Could you check a few things on this model? Use its own coordinates, in mm. Face numbers are marked on the shaded views. A direction names the side the tool comes from. Round coordinates to 2 decimals unless told otherwise and drop trailing zeros. Write each loop counter-clockwise with the first axis right and the second up, starting at its lowest first coordinate (ties: lowest second). Pieces come first, ordered by that corner, then holes. Notation, with made-up numbers: (18.25, 35) - (56.25, 35) arc R38 ccw to (56.25, 74) - close; hole circle Ø11 at (57, -13). An arc over 180 degrees is marked (long way). Write each question's results on one line, items separated by ' | '. Start each with the question number.
(1) Imagine slicing it at A-A on x = 0. Write out the boundary of the cut face in (y, z), then the cut area to 3 significant figures.
(2) Thinking about a two-plate mould opening in Y: for the marked faces 4, 5 and 6, which applies, +Y half, -Y half, draft (parallel to the pull), parting line (faces both ways), or undercut?
(3) Imagine slicing it at D-D on y = 7.5. Write out the boundary of the cut face in (x, z).
(4) For P1, Ø8, axis at y = -4.5, z = 9.5, coming from the -X side; P2, Ø1.5, axis at y = -8.5, z = 7.5, coming from the -X side; P3, Ø2.5, axis at x = -5.3, y = 5.3, coming from the +Z side; P4, Ø1.7, axis at x = 5.3, y = 5.3, coming from the -Z side, each with a flat end and sliding along its axis, tell me the tip position at first contact or that it passes through.
(5) Please list where these lines run through material, in increasing order: line 1 (Y direction, x = 0, z = 9.25); line 2 (X direction, y = 1.5, z = 7.25); line 3 (Y direction, x = 2.5, z = 13). Write a range as [from, to].
(6) Imagine slicing it at C-C on z = 15.25. Write out the boundary of the cut face in (x, y).
(7) On a 3-axis mill with a long thin cutter (end or side, diameter ignored), from which of +Z, -Z, +X, -X, +Y, -Y can I reach the whole of each face in a straight line? I mean the marked faces 1, 2 and 3. Say none if no direction works.
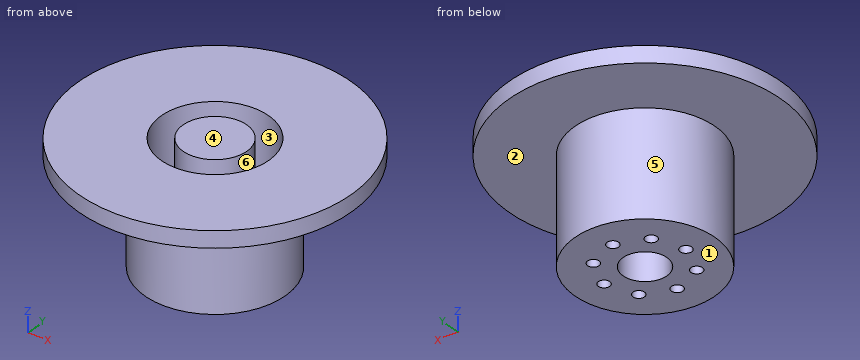
```python
from build123d import *

# Parameters (mm, degrees)
SKETCH4_R          = 1.05
CUT_EXTRUDE1_DEPTH = 4


with BuildPart() as part:
    # Sketch2 → Revolve1 (revolve)
    with BuildSketch(Plane(origin=(0, 0, 0), x_dir=(0, 0, -1), z_dir=(1, 0, 0))):
        Polygon((-22, 0), (-22, 5.8), (-3, 5.8), (-3, 9.8), (-22, 9.8), (-22, 24.8), (-19, 24.8), (-19, 12.8), (0, 12.8), (0, 4), (-19, 4), (-19, 0), align=None)
    revolve(axis=Axis((0, 0, 0), (0, 0, 1)))

    # Sketch4 → Cut-Extrude1 (cut, through all)
    with BuildSketch(Plane.XY.offset(3)):
        with Locations((0, 7.5)):
            Circle(SKETCH4_R)
        with Locations((5.303300859, 5.303300859)):
            Circle(SKETCH4_R)
        with Locations((7.5, 0)):
            Circle(SKETCH4_R)
        with Locations((5.303300859, -5.303300859)):
            Circle(SKETCH4_R)
        with Locations((0, -7.5)):
            Circle(SKETCH4_R)
        with Locations((-5.303300859, -5.303300859)):
            Circle(SKETCH4_R)
        with Locations((-7.5, 0)):
            Circle(SKETCH4_R)
        with Locations((-5.303300859, 5.303300859)):
            Circle(SKETCH4_R)
    extrude(amount=-CUT_EXTRUDE1_DEPTH, mode=Mode.SUBTRACT)


solid = part.part
```
Response:
1) outline: (-24.8, 19) - (-12.8, 19) - (-12.8, 0) - (-8.55, 0) - (-8.55, 3) - (-9.8, 3) - (-9.8, 22) - (-24.8, 22) - close; (-6.45, 0) - (-4, 0) - (-4, 19) - (4, 19) - (4, 0) - (6.45, 0) - (6.45, 3) - (5.8, 3) - (5.8, 22) - (-5.8, 22) - (-5.8, 3) - (-6.45, 3) - close; (8.55, 0) - (12.8, 0) - (12.8, 19) - (24.8, 19) - (24.8, 22) - (9.8, 22) - (9.8, 3) - (8.55, 3) - close | area: 319 mm²
2) face 4: draft | face 5: parting line | face 6: undercut
3) outline: (-23.64, 19) - (-10.37, 19) - (-10.37, 0) - (-1.05, 0) - (-1.05, 3) - (-6.31, 3) - (-6.31, 22) - (-23.64, 22) - close; (1.05, 0) - (10.37, 0) - (10.37, 19) - (23.64, 19) - (23.64, 22) - (6.31, 22) - (6.31, 3) - (1.05, 3) - close
4) P1: x = -12.79 | P2: x = -10.19 | P3: z = 3 | P4: through
5) line 1: [-12.8, -9.8], [-5.8, -4], [4, 5.8], [9.8, 12.8] | line 2: [-12.71, -9.68], [-5.6, -3.71], [3.71, 5.6], [9.68, 12.71] | line 3: [-12.55, -9.48], [-5.23, -3.12], [3.12, 5.23], [9.48, 12.55]
6) outline: circle Ø25.6 at (0, 0); circle Ø11.6 at (0, 0); hole circle Ø19.6 at (0, 0); hole circle Ø8 at (0, 0)
7) face 1: -Z, +X, -X, +Y, -Y | face 2: -Z | face 3: +Z
